For this review, take the finished solid that the model builds, in its own axes (mm). A direction names the side the tool comes from. Give positions to 0.01 mm unless a question says otherwise; leave off trailing zeros. Loops run counter-clockwise (first coordinate to the right, second up) from the corner with the lowest first, then second, coordinate; pieces in that order, holes last. Notation, with made-up numbers: (56, -2) -> (61, -2) arc R24 ccw to (61, 15) -> close; hole circle Ø8 at (-37, 2.5). An arc over 180 degrees is marked (long way). Answer as CSV lines item,"result". Start each with the question number.
Item 1: Add section B-B on z = -3. State the section outline as (x, y) points, plus the area to 3 significant figures.
Item 2: Machinability: for faces 1 (the face through (-304, -9.652, 0)), 2 (the face through (-304, -12.7, 0)), which of the approach directions +Z, -Z, +X, -X, +Y, -Y give a long, thin tool a straight path to every point of the face, cutting with its end or side? Answer none if there is none.
Item 3: For L1, parallel to Z at x = -43, y = -4.5; L2, parallel to Z at x = -380, y = -9.5, list the stretches that pass through material, from the lowest coordinate up. Write a range as from..to.
Item 4: Add section C-C on x = -486. State the section outline as (y, z) points, plus the area to 3 significant figures.
Item 5: The part is to be moulded in two halves that separate along Y. For faces 3 (the face through (-304, 12.7, 0)), 4 (the face through (-304, 0, -12.7)), 5 (the face through (-304, 0, -9.652)), say which applies: +Y half, -Y half, draft (parallel to the pull), parting line (faces both ways), or undercut.
Item 6: Add section A-A on y = -1. State the section outline as (x, z) points, plus the area to 3 significant figures.
```python
from build123d import *

# Parameters (mm, degrees)
SKETCH3_W           = 25.4
SKETCH3_H           = 25.4
SKETCH3_W_2         = 19.304
SKETCH3_H_2         = 19.304
BOSS_EXTRUDE1_DEPTH = 616.49
FILLET1_R           = 2.5
FILLET2_R           = 1
CUT_EXTRUDE1_DEPTH  = 618.143719161


with BuildPart() as part:
    # Sketch3 → Boss-Extrude1 (new body)
    with BuildSketch(Plane(origin=(0, 0, 0), x_dir=(0, 0, -1), z_dir=(1, 0, 0))):
        Rectangle(SKETCH3_W, SKETCH3_H)
        Rectangle(SKETCH3_W_2, SKETCH3_H_2, mode=Mode.SUBTRACT)
    extrude(amount=-BOSS_EXTRUDE1_DEPTH)

    # Fillet1
    fillet1_edges = [part.edges().sort_by_distance(p)[0] for p in [
        (-308.245, -12.7, -12.7),
        (-308.245, -12.7, 12.7),
        (-308.245, 12.7, 12.7),
        (-308.245, 12.7, -12.7),
    ]]
    fillet(fillet1_edges, radius=FILLET1_R)

    # Fillet2
    fillet2_edges = [part.edges().sort_by_distance(p)[0] for p in [
        (-308.245, 9.652, -9.652),
        (-308.245, -9.652, -9.652),
        (-308.245, -9.652, 9.652),
        (-308.245, 9.652, 9.652),
    ]]
    fillet(fillet2_edges, radius=FILLET2_R)

    # Sketch4 → Cut-Extrude1 (cut, through all)
    with BuildSketch(Plane.XY.offset(12.7)):
        Polygon((-616.49, 12.7), (-591.09, -12.7), (-616.49, -12.7), align=None)
        Polygon((0, 12.7), (-25.4, -12.7), (0, -12.7), align=None)
    extrude(amount=-CUT_EXTRUDE1_DEPTH, mode=Mode.SUBTRACT)


solid = part.part
```
Computed values:
1,outline,"(-616.49, 12.7) -> (-613.44, 9.65) -> (-3.05, 9.65) -> (0, 12.7) -> close; (-594.14, -9.65) -> (-591.09, -12.7) -> (-25.4, -12.7) -> (-22.35, -9.65) -> close"
1,area,"3,600 mm²"
2,face 1,"+X, -X"
2,face 2,"+Z, -Z, +X, -X, -Y"
3,L1,"-12.7..-9.65, 9.65..12.7"
3,L2,"-12.7..-9.18, 9.18..12.7"
4,outline,"(-12.7, -10.2) arc R2.5 ccw to (-10.2, -12.7) -> (10.2, -12.7) arc R2.5 ccw to (12.7, -10.2) -> (12.7, 10.2) arc R2.5 ccw to (10.2, 12.7) -> (-10.2, 12.7) arc R2.5 ccw to (-12.7, 10.2) -> close; hole (-9.65, -8.65) arc R1 ccw to (-8.65, -9.65) -> (8.65, -9.65) arc R1 ccw to (9.65, -8.65) -> (9.65, 8.65) arc R1 ccw to (8.65, 9.65) -> (-8.65, 9.65) arc R1 ccw to (-9.65, 8.65) -> close"
4,area,"268 mm²"
5,face 3,"+Y half"
5,face 4,"draft"
5,face 5,"undercut"
6,outline,"(-602.79, -12.7) -> (-13.7, -12.7) -> (-13.7, -9.65) -> (-602.79, -9.65) -> close; (-602.79, 9.65) -> (-13.7, 9.65) -> (-13.7, 12.7) -> (-602.79, 12.7) -> close"
6,area,"3,590 mm²"
